```python
from build123d import *

# Parameters (mm, degrees)
F2_R     = 7.9
F3_DEPTH = 2
F5_DEPTH = 2
F7_DEPTH = 1


with BuildPart() as f1:
    # F0 (on Front) → F1 (revolve)
    with BuildSketch(Plane.XZ):
        Polygon((2.5, 3.1889840401), (2.5, 0.6889840401), (9.5, 0.6889840401), (9.5, 1.1889840401), (7.5, 2.6889840401), (7.5, 3.1889840401), align=None)
    revolve(axis=Axis((0, 0, 1.9389840401), (0, 0, -1)))

    # F2 (on face) → F3 (join)
    with BuildSketch(Plane(origin=(0, 0, 0.6889840401), x_dir=(1, 0, 0), z_dir=(0, 0, -1))):
        Circle(F2_R)
    extrude(amount=F3_DEPTH)

    # F4 (on face) → F5 (cut)
    with BuildSketch(Plane(origin=(0, 0, -1.3110159599), x_dir=(1, 0, 0), z_dir=(0, 0, -1))):
        with BuildLine():
            ThreePointArc((2.1354156504, -1.3), (2.4071289045, -0.675078097), (2.5, 0))
            ThreePointArc((2.5, 0), (2.4071289045, 0.675078097), (2.1354156504, 1.3))
            Line((2.1354156504, 1.3), (-2.1354156504, 1.3))
            ThreePointArc((-2.1354156504, 1.3), (-2.5, 0), (-2.1354156504, -1.3))
            Line((-2.1354156504, -1.3), (2.1354156504, -1.3))
        make_face()
        with BuildLine():
            ThreePointArc((2.1354156504, 1.3), (2.4071289045, 0.675078097), (2.5, 0))
            ThreePointArc((2.5, 0), (2.4071289045, -0.675078097), (2.1354156504, -1.3))
            Line((2.1354156504, -1.3), (8.2728397101, -1.3))
            Line((8.2728397101, -1.3), (8.2728397101, 1.3))
            Line((8.2728397101, 1.3), (2.1354156504, 1.3))
        make_face()
        with BuildLine():
            Line((-2.1354156504, 1.3), (2.1354156504, 1.3))
            ThreePointArc((2.1354156504, 1.3), (0, 2.5), (-2.1354156504, 1.3))
        make_face()
        with BuildLine():
            ThreePointArc((-2.1354156504, -1.3), (0, -2.5), (2.1354156504, -1.3))
            Line((2.1354156504, -1.3), (-2.1354156504, -1.3))
        make_face()
        with BuildLine():
            ThreePointArc((-2.1354156504, -1.3), (-2.5, 0), (-2.1354156504, 1.3))
            Line((-2.1354156504, 1.3), (-8.2728397101, 1.3))
            Line((-8.2728397101, 1.3), (-8.2728397101, -1.3))
            Line((-8.2728397101, -1.3), (-2.1354156504, -1.3))
        make_face()
    extrude(amount=-F5_DEPTH, mode=Mode.SUBTRACT)

    # F6 (on face) → F7 (cut)
    with BuildSketch(Plane.XY.offset(3.1889840401)):
        with BuildLine():
            Line((0, -5.7335105867), (2.5289812019, -5.7335105867))
            ThreePointArc((2.5289812019, -5.7335105867), (0, 6.2664894133), (-2.5289812019, -5.7335105867))
            Line((-2.5289812019, -5.7335105867), (0, -5.7335105867))
        make_face()
    extrude(amount=-F7_DEPTH, mode=Mode.SUBTRACT)


solid = f1.part
```
Check sheet for the modelled part. Datum: model origin and axes. Units: mm. A direction names the side the tool comes from. Give positions to 0.01 mm unless a question says otherwise; leave off trailing zeros. Loops run counter-clockwise (first coordinate to the right, second up) from the corner with the lowest first, then second, coordinate; pieces in that order, holes last. Notation, with made-up numbers: (29, 22.25) - (41, 22.25) arc R16 cw to (41, 48.25) - close; hole circle Ø1 at (84, 51). An arc over 180 degrees is marked (long way). One line per question, with ' | ' between items. Start each with the question number.
1. Cross-section at D-D, the plane z = 1.75. Enter the section's corners in (x, y).
2. Material ranges on line 1 along Y through (x, z) = (0, 2.85); line 2 along X through (y, z) = (0, 2.9); line 3 along Z through (x, y) = (2.25, 3.75), recorded low to high. Write a range as [from, to].
3. Set-up check for faces 4 (the flat face through (0, -5.734, 3)), 5 (the flat face through (0, 5, -1.311)), 6 (the cylindrical face through (4.38, 8.43, 0.94)), 7 (the flat face through (-5, -1.3, 0)), 8 (the cylindrical face through (0.16, -7.9, -0.3)): record each of +Z, -Z, +X, -X, +Y, -Y from which the full face is reachable in a straight line by a thin tool's end or side.
4. Cross-section at C-C, the plane x = 0. Enter the section's corners in (y, z).
5. Cross-section at B-B, the plane y = 0. Enter the section's corners in (x, z), plus the area to 3 significant figures.
6. Draft check along Y on faces 1 (the flat face through (0, -6, 3.189)), 2 (the flat face through (-5, 1.3, 0)), 3 (the cylindrical face through (-0.16, 7.9, -0.3)). Enter one of: released by +Y, released by -Y, zero draft, split by the parting line, or undercut.
7. Gauge pin test, flat ends, axial feed: pin 1 Ø1.5 at (x, z) = (-3, 1.5) entering from -Y; pin 2 Ø1.6 at (x, z) = (-5, 0) entering from -Y; pin 3 Ø2 at (x, z) = (5, -0.5) entering from +Y. Record the tip position at first contact, or that the pin passes through.
8. Cross-section at A-A, the plane z = 0.25. Enter the section's corners in (x, y).
Check result:
1) outline: circle Ø17.5 at (0, 0); hole circle Ø5 at (0, 0)
2) line 1: y = [-7.5, -5.73], [6.27, 7.5] | line 2: x = [-7.5, -6.27], [6.27, 7.5] | line 3: z = [-1.31, 2.19]
3) face 4: +Z | face 5: -Z, +X, -X, +Y, -Y | face 6: +Z, -Z | face 7: -Z, +X, -X | face 8: -Z, -Y
4) outline: (-9.5, 0.69) - (-7.9, 0.69) - (-7.9, -1.31) - (-2.5, -1.31) - (-2.5, 2.19) - (-5.73, 2.19) - (-5.73, 3.19) - (-7.5, 3.19) - (-7.5, 2.69) - (-9.5, 1.19) - close; (2.5, -1.31) - (7.9, -1.31) - (7.9, 0.69) - (9.5, 0.69) - (9.5, 1.19) - (7.5, 2.69) - (7.5, 3.19) - (6.27, 3.19) - (6.27, 2.19) - (2.5, 2.19) - close
5) outline: (-9.5, 0.69) - (-2.5, 0.69) - (-2.5, 2.19) - (-6.27, 2.19) - (-6.27, 3.19) - (-7.5, 3.19) - (-7.5, 2.69) - (-9.5, 1.19) - close; (2.5, 0.69) - (9.5, 0.69) - (9.5, 1.19) - (7.5, 2.69) - (7.5, 3.19) - (6.27, 3.19) - (6.27, 2.19) - (2.5, 2.19) - close | area: 22.5 mm2
6) face 1: zero draft | face 2: undercut | face 3: released by +Y
7) pin 1: stops at y = -9.21 | pin 2: stops at y = -8.32 | pin 3: stops at y = 6.81
8) outline: (-7.79, -1.3) arc R7.9 ccw to (7.79, -1.3) - (2.14, -1.3) arc R2.5 cw to (-2.14, -1.3) - close; (-7.79, 1.3) - (-2.14, 1.3) arc R2.5 cw to (2.14, 1.3) - (7.79, 1.3) arc R7.9 ccw to start
